from build123d import *

# Parameters (mm, degrees)
BOSS_EXTRUDE1_DEPTH = 88.9
SKETCH2_R           = 3.175
CUT_EXTRUDE1_DEPTH  = 4.175
FILLET1_R           = 6.35


with BuildPart() as part:
    # Sketch1 → Boss-Extrude1 (new body)
    with BuildSketch(Plane.XY):
        with BuildLine():
            Line((13.335, 323.089397322), (10.16, 323.089397322))
            Line((10.16, 323.089397322), (10.16, 288.164397322))
            Line((10.16, 288.164397322), (19.685, 288.164397322))
            ThreePointArc((19.685, 288.164397322), (29.21, 278.639397322), (19.685, 269.114397322))
            Line((19.685, 269.114397322), (10.16, 269.114397322))
            Line((10.16, 269.114397322), (10.16, 234.189397322))
            Line((10.16, 234.189397322), (13.335, 234.189397322))
            Line((13.335, 234.189397322), (13.335, 265.939397322))
            Line((13.335, 265.939397322), (19.685, 265.939397322))
            ThreePointArc((19.685, 265.939397322), (32.385, 278.639397322), (19.685, 291.339397322))
            Line((19.685, 291.339397322), (13.335, 291.339397322))
            Line((13.335, 291.339397322), (13.335, 323.089397322))
        make_face()
    extrude(amount=-BOSS_EXTRUDE1_DEPTH)

    # Sketch2 → Cut-Extrude1 (cut, through all)
    with BuildSketch(Plane(origin=(13.335, 0, 0), x_dir=(0, 0, -1), z_dir=(1, 0, 0))):
        with Locations((41.275, 250.064397322)):
            Circle(SKETCH2_R)
        with Locations((76.2, 250.064397322)):
            Circle(SKETCH2_R)
        with Locations((76.2, 307.214397322)):
            Circle(SKETCH2_R)
        with Locations((41.275, 307.214397322)):
            Circle(SKETCH2_R)
    extrude(amount=-CUT_EXTRUDE1_DEPTH, mode=Mode.SUBTRACT)

    # Fillet1
    fillet1_edges = [part.edges().sort_by_distance(p)[0] for p in [
        (11.7475, 323.089397322, 0),
        (11.7475, 234.189397322, 0),
        (11.7475, 234.189397322, -88.9),
        (11.7475, 323.089397322, -88.9),
    ]]
    fillet(fillet1_edges, radius=FILLET1_R)


solid = part.part
Verification items for the finished model (mm, model axes). A direction names the side the tool comes from. Coordinates: 2 decimals unless noted, no trailing zeros. Write each loop counter-clockwise with the first axis right and the second up, starting at its lowest first coordinate (ties: lowest second). Pieces come first, ordered by that corner, then holes. Notation, with made-up numbers: M -32,27 L 19,27 A27 cw 19,52 Z; hole C 22,2.5 d2. An arc over 180 degrees is marked long. Use CSV: the item, a comma, the result in double quotes.
Q1. Section check B-B, the plane x = 16.75. Enter the section's corners in (y, z).
Computed values:
outline,"M 265.94,-88.9 L 269.11,-88.9 L 269.11,0 L 265.94,0 Z; M 288.16,-88.9 L 291.34,-88.9 L 291.34,0 L 288.16,0 Z"
Q2. Thickness scan on line 1 along Y through (x, z) = (11.65, -76.2); line 2 along Y through (x, z) = (16, -23.5); line 3 along Y through (x, z) = (12.75, -54). Record the ranges inside material, lowest first. Write a range as [from, to].
Computed values:
line 1,"[234.19, 246.89], [253.24, 269.11], [288.16, 304.04], [310.39, 323.09]"
line 2,"[265.94, 269.11], [288.16, 291.34]"
line 3,"[234.19, 269.11], [288.16, 323.09]"
Q3. Mould release check, pull along Y, two halves, no side actions. Record for faces 1 (the flat face through (25, 270, 0)), 2 (the flat face through (12, 234.189, -44)), 3 (the flat face through (15, 269.114, -44)): pulls with the +Y half, pulls with the -Y half, needs draft (parallel to the pull), parting line crosses it, or undercut.
Computed values:
face 1,"needs draft"
face 2,"pulls with the -Y half"
face 3,"undercut"
Q4. Set-up check for faces 4 (the flat face through (13.335, 246, -44)), 5 (the flat face through (17, 291.339, -44)), 6 (the flat face through (25, 270, -88.9)): record each of +Z, -Z, +X, -X, +Y, -Y from which the full face is reachable in a straight line by a thin tool's end or side.
Computed values:
face 4,"+Z, -Z, +X, -Y"
face 5,"+Z, -Z, +X, +Y"
face 6,"-Z, +X, -X, +Y, -Y"
Q5. Section check C-C, the plane y = 249. Enter the section's corners in (x, z) (3 decimals), and give its area (3 significant figures).
Computed values:
outline,"M 10.16,-88.9 L 13.335,-88.9 L 13.335,-79.191 L 10.16,-79.191 Z; M 10.16,-73.209 L 13.335,-73.209 L 13.335,-44.266 L 10.16,-44.266 Z; M 10.16,-38.284 L 13.335,-38.284 L 13.335,0 L 10.16,0 Z"
area,"244 mm²"
Q6. Go/stop test with flat-tipped pins: P1, Ø3, axis at x = 16, z = -37, coming from the +Y side; P2, Ø4, axis at x = 25.5, z = -41, coming from the -Y side; P3, Ø7.5, axis at y = 250.06, z = -41.28, coming from the +X side (3 decimals). Record where each tip stops, or that it passes through.
Computed values:
P1,"y = 291.34"
P2,"y = 266.53"
P3,"x = 13.335"
Q7. Section check A-A, the plane z = -76.2. Enter the section's corners in (x, y) (3 decimals), and give its area (3 significant figures).
Computed values:
outline,"M 10.16,234.189 L 13.335,234.189 L 13.335,246.889 L 10.16,246.889 Z; M 10.16,253.239 L 13.335,253.239 L 13.335,265.939 L 19.685,265.939 A12.7 ccw 19.685,291.339 L 13.335,291.339 L 13.335,304.039 L 10.16,304.039 L 10.16,288.164 L 19.685,288.164 A9.525 cw 19.685,269.114 L 10.16,269.114 Z; M 10.16,310.389 L 13.335,310.389 L 13.335,323.089 L 10.16,323.089 Z"
area,"333 mm²"
Q8. Section check D-D, the plane z = -59.5. Enter the section's corners in (x, y) (3 decimals).
Computed values:
outline,"M 10.16,234.189 L 13.335,234.189 L 13.335,265.939 L 19.685,265.939 A12.7 ccw 19.685,291.339 L 13.335,291.339 L 13.335,323.089 L 10.16,323.089 L 10.16,288.164 L 19.685,288.164 A9.525 cw 19.685,269.114 L 10.16,269.114 Z"
